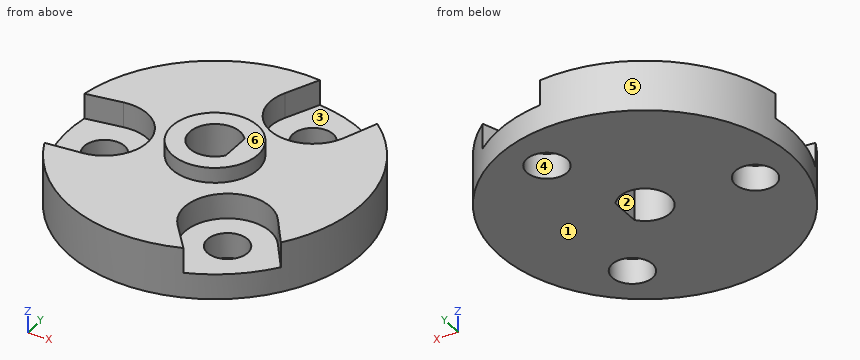
from build123d import *

# Parameters (mm, degrees)
SKETCH034_R          = 14.5
PAD014_DEPTH         = 5
SKETCH035_R          = 4.25
PAD015_DEPTH         = 1.5
SKETCH036_R          = 2
POCKET019_DEPTH      = 88.049178788
POCKET020_DEPTH      = 2.5
POLARPATTERN_COUNT   = 3
POCKET021_DEPTH      = 5.001
POCKET021_DEPTH_BACK = 1.501


with BuildPart() as part:
    # Sketch034 → Pad014 (new body)
    with BuildSketch(Plane.XY.offset(40.1)):
        Circle(SKETCH034_R)
    extrude(amount=PAD014_DEPTH)

    # Sketch035 → Pad015 (join)
    with BuildSketch(Plane.XY.offset(45.1)):
        Circle(SKETCH035_R)
    extrude(amount=PAD015_DEPTH)

    # Sketch036 → Pocket019 (cut, through all)
    with BuildSketch(Plane.XY.offset(45.1)):
        with Locations((-10.0992623493, -1.43)):
            Circle(SKETCH036_R)
    pocket019 = extrude(amount=-POCKET019_DEPTH, mode=Mode.SUBTRACT)

    # Sketch037 → Pocket020 (cut)
    with BuildSketch(Plane.XY.offset(45.1)):
        with BuildLine():
            ThreePointArc((-9.644040596, -5.6555500417), (-5.8912363704, -0.8341666667), (-10.83504492, 2.7558241732))
            Line((-10.83504492, 2.7558241732), (-14.3412882274, 2.1394980669))
            ThreePointArc((-14.3412882274, 2.1394980669), (-14.3567945162, -2.0328431373), (-13.1835601604, -6.0368652045))
            Line((-9.644040596, -5.6555500417), (-13.1835601604, -6.0368652045))
        make_face()
    pocket020 = extrude(amount=-POCKET020_DEPTH, mode=Mode.SUBTRACT)

    # PolarPattern: Pocket019, Pocket020 ×3 about axis
    polarpattern_axis = Axis((0, 0, 45.1), (0, 0, 1))
    for i in range(1, POLARPATTERN_COUNT):
        add(pocket019.rotate(polarpattern_axis, i * 360 / POLARPATTERN_COUNT), mode=Mode.SUBTRACT)
        add(pocket020.rotate(polarpattern_axis, i * 360 / POLARPATTERN_COUNT), mode=Mode.SUBTRACT)

    # Sketch038 → Pocket021 (cut, two sides)
    with BuildSketch(Plane.XY.offset(45.1)) as pocket021_sk:
        with BuildLine():
            Line((2, 1.5), (2, -1.5))
            ThreePointArc((2, 1.5), (-2.5, 0), (2, -1.5))
        make_face()
    extrude(amount=-POCKET021_DEPTH, mode=Mode.SUBTRACT)
    extrude(pocket021_sk.sketch, amount=POCKET021_DEPTH_BACK, mode=Mode.SUBTRACT)


solid = part.part
Can you work these out from the model? Positions are in its coordinate system, mm. Face numbers are marked on the shaded views. A direction names the side the tool comes from. Coordinates: 2 decimals unless noted, no trailing zeros. Order: outer loops, then holes, each group sorted by start corner. A loop starts at its lowest first (then second) coordinate and runs counter-clockwise, first axis right, second up. Notation, with made-up numbers: M 72.25,-29.5 L 86.25,-29.5 A34 ccw 86.25,8.5 Z; hole C 81,38.5 d7. An arc over 180 degrees is marked long. Write item = value, one per line.
(1) Suppose I cut it at C-C on y = 6. Please give me the cut outline in (x, z).
Results are:
outline = M -13.2,40.1 L 13.2,40.1 L 13.2,45.1 L 6.28,45.1 L 6.28,42.6 L 1.34,42.6 L 1.34,45.1 L -13.2,45.1 Z
(2) Suppose I cut it at B-B on y = 0. Please give me the cut outline in (x, z), plus the area to 3 significant figures.
Results are:
outline = M -14.5,40.1 L -11.5,40.1 L -11.5,42.6 L -14.5,42.6 Z; M -8.7,40.1 L -2.5,40.1 L -2.5,46.6 L -4.25,46.6 L -4.25,45.1 L -6.1,45.1 L -6.1,42.6 L -8.7,42.6 Z; M 2,40.1 L 14.5,40.1 L 14.5,45.1 L 4.25,45.1 L 4.25,46.6 L 2,46.6 Z
area = 101 mm2
(3) I need wall thicknesses on line 1 along Y through (x, z) = (0, 42); line 2 along Y through (x, z) = (0, 42.75); line 3 along X through (y, z) = (-0.5, 41). Which ranges of each line are inside material? Lowest first, please. Write a range as [from, to].
Results are:
line_1 = [-14.5, -2.5], [2.5, 14.5]
line_2 = [-14.5, -2.5], [2.5, 7.58], [11.35, 14.5]
line_3 = [-14.49, -11.87], [-8.33, -2.45], [2, 14.49]
(4) Suppose I cut it at A-A on z = 43.75. Please give me the cut outline in (x, y), plus the area to 3 significant figures.
Results are:
outline = M -14.34,2.14 L -10.84,2.76 A4.25 cw long -9.64,-5.66 L -13.18,-6.04 A14.5 ccw 5.32,-13.49 L 3.03,-10.76 A4.25 cw long 9.72,-5.52 L 11.82,-8.4 A14.5 ccw 9.02,11.35 L 7.8,8.01 A4.25 cw long -0.08,11.18 L 1.36,14.44 A14.5 ccw Z; hole M 2,-1.5 L 2,1.5 A2.5 ccw long Z
area = 454 mm2
(5) For pin 1 Ø4.5 at (x, y) = (-10.1, -1.43) entering from +Z; pin 2 Ø3 at (x, y) = (-11.5, 8.5) entering from +Z; pin 3 Ø1.5 at (x, z) = (-9, 43) entering from +Y, each with a flat end and sliding along its axis, tell me the tip position at first contact or that it passes through.
Results are:
pin_1 = 42.6
pin_2 = 45.1
pin_3 = 11.92
(6) If we mould it in two halves opening along X, with no side actions, what happens to the marked faces 4, 5 and 6? For each: pulls with the +X half, pulls with the -X half, needs draft (parallel to the pull), parting line crosses it, or undercut.
Results are:
face_4 = undercut
face_5 = parting line crosses it
face_6 = needs draft
(7) For the marked faces 1, 2 and 3, which set-ups out of +Z, -Z, +X, -X, +Y, -Y let a thin tool reach every point of the face, with its end or its side?
Results are:
face_1 = -Z, +X, -X, +Y, -Y
face_2 = +Z, -Z
face_3 = +Z
